from build123d import *

# Parameters (mm, degrees)
SKETCH_1_R               = 40.028115119
EXTRUDE_1_DEPTH          = 3
CHAMFER_1_SIZE           = 1
CUT_EXTRUDE_1_DEPTH      = 294.143309663
CUT_EXTRUDE_1_DEPTH_BACK = 294.143309663
SKETCH_2_R               = 2.5
CUT_EXTRUDE_2_DEPTH      = 294.143309663
CUT_EXTRUDE_2_DEPTH_BACK = 294.143309663
SKETCH_3_R               = 10.25
CUT_EXTRUDE_3_DEPTH      = 294.143309663
CUT_EXTRUDE_3_DEPTH_BACK = 294.143309663
SKETCH_4_R               = 1.5
CUT_EXTRUDE_4_DEPTH      = 294.143309663
CUT_EXTRUDE_4_DEPTH_BACK = 294.143309663
SKETCH_5_R               = 1.5
CUT_EXTRUDE_5_DEPTH      = 294.143309663
CUT_EXTRUDE_5_DEPTH_BACK = 294.143309663
SKETCH_6_R               = 1.5


with BuildPart() as part:
    # 草图1 → 凸台-拉伸1 (new body)
    with BuildSketch(Plane.XY):
        with BuildLine():
            Line((44.764783638, 38.458868953), (4.334015044, 74.86289651))
            ThreePointArc((4.334015044, 74.86289651), (-1.881238093, 78.67160853), (-9.048597084, 80))
            Line((-9.048597084, 80), (-225.951402916, 80))
            ThreePointArc((-225.951402916, 80), (-233.118761907, 78.67160853), (-239.334015044, 74.86289651))
            Line((-239.334015044, 74.86289651), (-279.764783638, 38.458868953))
            ThreePointArc((-279.764783638, 38.458868953), (-281.748934241, 33.886916076), (-279.593885752, 29.392989871))
            ThreePointArc((-279.593885752, 29.392989871), (-276.958783906, 25.06173547), (-277.521429039, 20.023188369))
            ThreePointArc((-277.521429039, 20.023188369), (-282, 0), (-277.521429039, -20.023188369))
            ThreePointArc((-277.521429039, -20.023188369), (-276.958783906, -25.06173547), (-279.593885752, -29.392989871))
            ThreePointArc((-279.593885752, -29.392989871), (-281.657387183, -32.949868258), (-280.946152423, -37))
            Line((-280.946152423, -37), (-274.883974596, -47.5))
            ThreePointArc((-274.883974596, -47.5), (-269.393593539, -52.990381057), (-261.893593539, -55))
            Line((-261.893593539, -55), (26.893593539, -55))
            ThreePointArc((26.893593539, -55), (34.393593539, -52.990381057), (39.883974596, -47.5))
            Line((39.883974596, -47.5), (45.946152423, -37))
            ThreePointArc((45.946152423, -37), (46.657387183, -32.949868258), (44.593885752, -29.392989871))
            ThreePointArc((44.593885752, -29.392989871), (41.958783906, -25.06173547), (42.521429039, -20.023188369))
            ThreePointArc((42.521429039, -20.023188369), (47, 0), (42.521429039, 20.023188369))
            ThreePointArc((42.521429039, 20.023188369), (41.958783906, 25.06173547), (44.593885752, 29.392989871))
            ThreePointArc((44.593885752, 29.392989871), (46.748934241, 33.886916076), (44.764783638, 38.458868953))
        make_face()
        with Locations(Location((0, 0, 0), (0, 0, 180))):
            Circle(SKETCH_1_R, mode=Mode.SUBTRACT)
        with Locations(Location((-235, 0, 0), (0, 0, 180))):
            Circle(SKETCH_1_R, mode=Mode.SUBTRACT)
    extrude(amount=EXTRUDE_1_DEPTH)

    # 倒角1
    chamfer_1_edges = [part.edges().sort_by_distance(p)[0] for p in [
        (40.028115119, 0, 3),
        (-194.971884881, 0, 3),
    ]]
    chamfer(chamfer_1_edges, length=CHAMFER_1_SIZE)

    # 草图2 → 切除-拉伸1 (cut, two sides: drawn at the far end of the back side and taken through both)
    with BuildSketch(Plane(origin=(0, 0, 0), x_dir=(-1, 0, 0), z_dir=(0, 0, -1)).offset(-CUT_EXTRUDE_1_DEPTH_BACK)):
        with Locations((40.75, -34)):
            Circle(SKETCH_2_R)
        with Locations((40.75, 34)):
            Circle(SKETCH_2_R)
        with Locations((-40.75, 34)):
            Circle(SKETCH_2_R)
        with Locations((-40.75, -34)):
            Circle(SKETCH_2_R)
        with Locations((275.75, -34)):
            Circle(SKETCH_2_R)
        with Locations((275.75, 34)):
            Circle(SKETCH_2_R)
        with Locations((194.25, 34)):
            Circle(SKETCH_2_R)
        with Locations((194.25, -34)):
            Circle(SKETCH_2_R)
    extrude(amount=CUT_EXTRUDE_1_DEPTH + CUT_EXTRUDE_1_DEPTH_BACK, mode=Mode.SUBTRACT)

    # 草图3 → 切除-拉伸2 (cut, two sides: drawn at the far end of the back side and taken through both)
    with BuildSketch(Plane.XY.offset(3).offset(-CUT_EXTRUDE_2_DEPTH_BACK)):
        with Locations((-117.5, -35)):
            Circle(SKETCH_3_R)
        with Locations((-225.951402916, 60)):
            Circle(SKETCH_3_R)
        with Locations((-117.5, 60)):
            Circle(SKETCH_3_R)
        with Locations((-9.048597084, 60)):
            Circle(SKETCH_3_R)
    extrude(amount=CUT_EXTRUDE_2_DEPTH + CUT_EXTRUDE_2_DEPTH_BACK, mode=Mode.SUBTRACT)

    # 草图4 → 切除-拉伸3 (cut, two sides: drawn at the far end of the back side and taken through both)
    with BuildSketch(Plane(origin=(0, 0, 0), x_dir=(-1, 0, 0), z_dir=(0, 0, -1)).offset(-CUT_EXTRUDE_3_DEPTH_BACK)):
        with Locations((134, -24.75)):
            Circle(SKETCH_4_R)
        with Locations((134, -45.25)):
            Circle(SKETCH_4_R)
        with Locations((101, -45.25)):
            Circle(SKETCH_4_R)
        with Locations((101, -24.75)):
            Circle(SKETCH_4_R)
    extrude(amount=CUT_EXTRUDE_3_DEPTH + CUT_EXTRUDE_3_DEPTH_BACK, mode=Mode.SUBTRACT)

    # 草图5 → 切除-拉伸4 (cut, two sides: drawn at the far end of the back side and taken through both)
    with BuildSketch(Plane(origin=(0, 0, 0), x_dir=(-1, 0, 0), z_dir=(0, 0, -1)).offset(-CUT_EXTRUDE_4_DEPTH_BACK)):
        with Locations((19.128165824, 48.891341485)):
            Circle(SKETCH_5_R)
        with Locations((25.048597084, 60)):
            Circle(SKETCH_5_R)
        with Locations((25.048597084, 76)):
            Circle(SKETCH_5_R)
        with Locations((3.314709891, 74.937286824)):
            Circle(SKETCH_5_R)
        with Locations((-13.547809826, 61.184227506)):
            Circle(SKETCH_5_R)
        with Locations((-4.229232955, 52.329375962)):
            Circle(SKETCH_5_R)
        with Locations((209.951402916, 60)):
            Circle(SKETCH_5_R)
        with Locations((215.871834176, 48.891341485)):
            Circle(SKETCH_5_R)
        with Locations((239.229232955, 52.329375962)):
            Circle(SKETCH_5_R)
        with Locations((248.547809826, 61.184227506)):
            Circle(SKETCH_5_R)
        with Locations((209.951402916, 76)):
            Circle(SKETCH_5_R)
        with Locations((231.685290109, 74.937286824)):
            Circle(SKETCH_5_R)
    extrude(amount=CUT_EXTRUDE_4_DEPTH + CUT_EXTRUDE_4_DEPTH_BACK, mode=Mode.SUBTRACT)

    # 草图6 → 切除-拉伸5 (cut, two sides: drawn at the far end of the back side and taken through both)
    with BuildSketch(Plane(origin=(0, 0, 0), x_dir=(-1, 0, 0), z_dir=(0, 0, -1)).offset(-CUT_EXTRUDE_5_DEPTH_BACK)):
        with Locations((134, 70.25)):
            Circle(SKETCH_6_R)
        with Locations((134, 49.75)):
            Circle(SKETCH_6_R)
        with Locations((101, 70.25)):
            Circle(SKETCH_6_R)
        with Locations((101, 49.75)):
            Circle(SKETCH_6_R)
    extrude(amount=CUT_EXTRUDE_5_DEPTH + CUT_EXTRUDE_5_DEPTH_BACK, mode=Mode.SUBTRACT)


solid = part.part
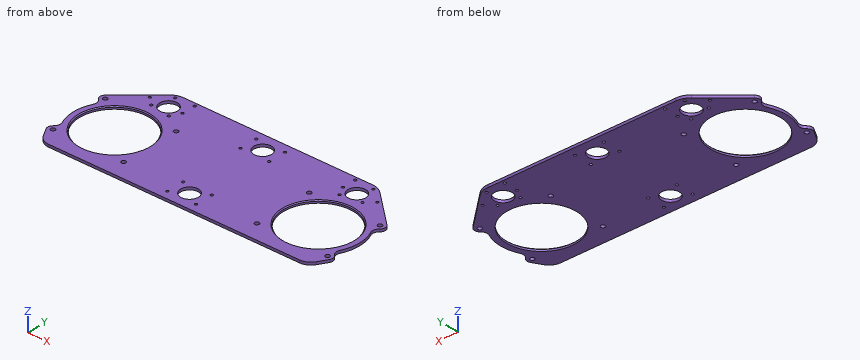
Read the model definition and answer for the solid it produces. Units are mm, in the model's axes. Give positions to 0.01 mm unless a question says otherwise; leave off trailing zeros. Write each loop counter-clockwise with the first axis right and the second up, starting at its lowest first coordinate (ties: lowest second). Pieces come first, ordered by that corner, then holes. Notation, with made-up numbers: (-10.75, -32) - (5.25, -32) arc R15 cw to (5.25, -13) - close; hole circle Ø5 at (-28, -31.75). An arc over 180 degrees is marked (long way). Answer in a Markdown table with one row per item. Add a question column.
Item 1: A flat-ended cylindrical pin translates along its axis: P1, Ø2.5, axis at x = -134, y = -45.25, coming from the +Z side. Find the tip coordinate at first contact, or state that the pin passes through.
Item 2: Find the intervals of material crossed by L1, parallel to Y at x = -101, z = 1; L2, parallel to Y at x = -117.5, z = 1.6; L3, parallel to X at y = -45.5, z = 0.15, in increasing order.
Item 3: Section B-B, the plane y = 26 is taken. Count the separate pieces of the cut face and the enclosed holes in it, and give its area (3 significant figures).
Item 4: Section A-A, the plane x = -117.5 is taken. Write down the section's boundary in (y, z).
Recorded:
| question | item | result |
|---|---|---|
| 1 | P1 | passes through |
| 2 | L1 | y = -55 to -46.75, -43.75 to -26.25, -23.25 to 48.25, 51.25 to 68.75, 71.75 to 80 |
| 2 | L2 | y = -55 to -45.25, -24.75 to 49.75, 70.25 to 80 |
| 2 | L3 | x = -276.04 to -135.48, -132.52 to -102.48, -99.52 to 41.04 |
| 3 | separate pieces | 3 |
| 3 | enclosed holes | 0 |
| 3 | area | 591 mm2 |
| 4 | outline | (-55, 0) - (-45.25, 0) - (-45.25, 3) - (-55, 3) - close; (-24.75, 0) - (49.75, 0) - (49.75, 3) - (-24.75, 3) - close; (70.25, 0) - (80, 0) - (80, 3) - (70.25, 3) - close |
